The figure shows three views and two pictorial views of one solid part (mm, origin at its lowest corner). Answer the questions. A direction names the side the tool comes from. Coordinates: 2 decimals unless noted, no trailing zeros. Write each loop counter-clockwise with the first axis right and the second up, starting at its lowest first coordinate (ties: lowest second). Pieces come first, ordered by that corner, then holes. Notation, with made-up numbers: M -35.75,-15 L -12.75,-15 A24 ccw -12.75,21 Z; hole C 7,-40 d7. An arc over 180 degrees is marked long. Use CSV: the item, a comma, the result in double quotes.
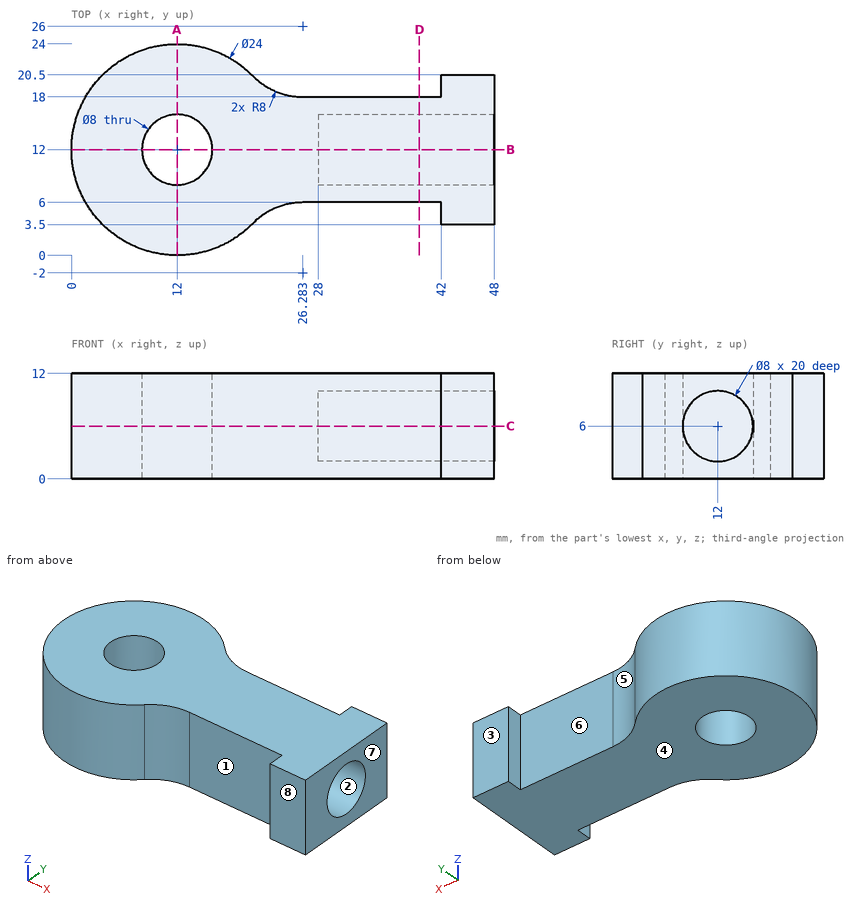
Item 1: The part is cut by section D-D (x = 39.5). Write down the section's boundary in (y, z).
Answer:
outline,"M 6,0 L 18,0 L 18,12 L 6,12 Z; hole C 12,6 d8"
Item 2: Consider probe 1 along Z at (x, y) = (33.25, 12); probe 2 along Y at (x, z) = (39.5, 6); probe 3 along X at (y, z) = (12, 6.5). Determine where each line is inside the solid, lowest interval first.
Answer:
probe 1,"z = 0 to 2, 10 to 12"
probe 2,"y = 6 to 8, 16 to 18"
probe 3,"x = 0 to 8, 16 to 28"
Item 3: The part is cut by section A-A (x = 12). Write down the section's boundary in (y, z), then the cut area to 3 significant figures.
Answer:
outline,"M 0,0 L 8,0 L 8,12 L 0,12 Z; M 16,0 L 24,0 L 24,12 L 16,12 Z"
area,"192 mm2"
Item 4: For a pull along X with two mould halves and no side action, classify the marked faces 6, 7 and 8 as released by +X, released by -X, zero draft, split by the parting line, or undercut.
Answer:
face 6,"undercut"
face 7,"released by +X"
face 8,"zero draft"
Item 5: Given pin 1 (2 mm diameter, centred on y = 4.5, z = 4.5, fed in from -X); pin 2 (6.5 mm diameter, centred on x = 45.5, z = 7, fed in from -Y); pin 3 (6 mm diameter, centred on x = 36, z = 5.5, fed in from +Y), each flat-ended and moving along its own axis, determine where each tip first touches the part or whether it passes through.
Answer:
pin 1,"stops at x = 1.91"
pin 2,"stops at y = 3.5"
pin 3,"stops at y = 18"
Item 6: The part is cut by section C-C (z = 6). Write down the section's boundary in (x, y).
Answer:
outline,"M 20.57,3.6 A8 cw 26.28,6 L 42,6 L 42,3.5 L 48,3.5 L 48,8 L 28,8 L 28,16 L 48,16 L 48,20.5 L 42,20.5 L 42,18 L 26.28,18 A8 cw 20.57,20.4 A12 ccw long Z; hole C 12,12 d8"
Item 7: The part is cut by section B-B (y = 12). Write down the section's boundary in (x, z).
Answer:
outline,"M 0,0 L 8,0 L 8,12 L 0,12 Z; M 16,0 L 48,0 L 48,2 L 28,2 L 28,10 L 48,10 L 48,12 L 16,12 Z"
Item 8: A tool of negligible diameter and unlimited length cuts with its end or side. For the marked faces 1, 2, 3, 4 and 5, from which of +Z, -Z, +X, -X, +Y, -Y can it reach the whole face along a straight path? Write none if from no direction.
Answer:
face 1,"+Z, -Z, -Y"
face 2,"+X"
face 3,"+Z, -Z, +X, +Y"
face 4,"-Z, +X, -X, +Y, -Y"
face 5,"+Z, -Z, +Y"
